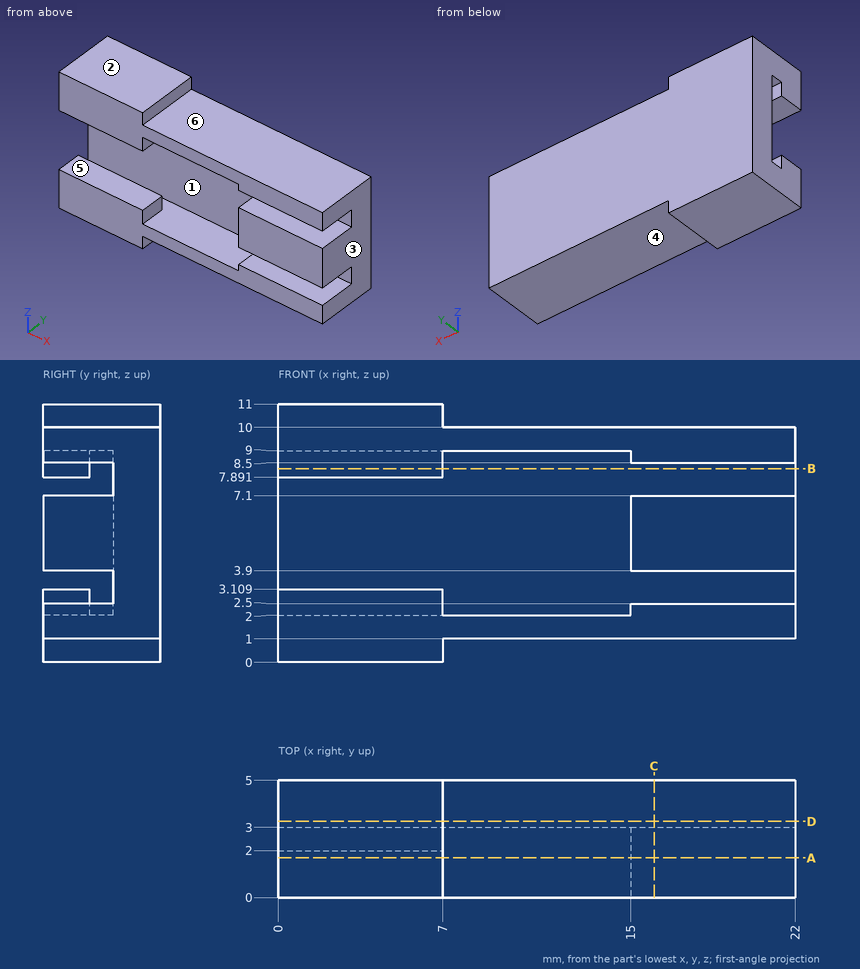
Input: dimensioned drawing with shaded views. Units: mm. Origin: part minimum x, y, z. A direction names the side the tool comes from. Coordinates: 2 decimals unless noted, no trailing zeros. Order: outer loops, then holes, each group sorted by start corner. A loop starts at its lowest first (then second) coordinate and runs counter-clockwise, first axis right, second up. Notation, with made-up numbers: (-10, -25) -> (3, -25) arc R32 cw to (3, 1) -> close; hole circle Ø9 at (31, 56). An arc over 180 degrees is marked (long way). Answer in a Markdown table with one row per item.
Item 1: Section B-B on z = 8.25. Output: boundary loops of the cut face in (x, y), plus the area to 3 significant figures.
Return value:
| item | result |
|---|---|
| outline | (0, 0) -> (7, 0) -> (7, 2) -> (0, 2) -> close; (0, 3) -> (22, 3) -> (22, 5) -> (0, 5) -> close |
| area | 58.0 mm² |
Item 2: Section D-D on y = 3.25. Output: boundary loops of the cut face in (x, z).
Return value:
| item | result |
|---|---|
| outline | (0, 0) -> (7, 0) -> (7, 1) -> (22, 1) -> (22, 10) -> (7, 10) -> (7, 11) -> (0, 11) -> close |
Item 3: Section A-A on y = 1.7. Output: boundary loops of the cut face in (x, z).
Return value:
| item | result |
|---|---|
| outline | (0, 0) -> (7, 0) -> (7, 1) -> (22, 1) -> (22, 2.5) -> (15, 2.5) -> (15, 2) -> (7, 2) -> (7, 3.11) -> (0, 3.11) -> close; (0, 7.89) -> (7, 7.89) -> (7, 9) -> (15, 9) -> (15, 8.5) -> (22, 8.5) -> (22, 10) -> (7, 10) -> (7, 11) -> (0, 11) -> close; (15, 3.9) -> (22, 3.9) -> (22, 7.1) -> (15, 7.1) -> close |
Item 4: Access query for the marked faces 4, 5 and 6. Directions: +Z, -Z, +X, -X, +Y, -Y. A direction counts if a zero-diameter tool reaches every point of the face in a straight line with its end or side. Return the directions, or none.
Return value:
| item | result |
|---|---|
| face 4 | -Z, +X, +Y, -Y |
| face 5 | +X, -X, -Y |
| face 6 | +Z, +X, +Y, -Y |
Item 5: Section C-C on x = 16. Output: boundary loops of the cut face in (y, z).
Return value:
| item | result |
|---|---|
| outline | (0, 1) -> (5, 1) -> (5, 10) -> (0, 10) -> (0, 8.5) -> (3, 8.5) -> (3, 7.1) -> (0, 7.1) -> (0, 3.9) -> (3, 3.9) -> (3, 2.5) -> (0, 2.5) -> close |
Item 6: Draft query along Z for the marked faces 1, 2 and 3. Return one class per face: released by +Z, released by -Z, zero draft, split by the parting line, or undercut.
Return value:
| item | result |
|---|---|
| face 1 | undercut |
| face 2 | released by +Z |
| face 3 | zero draft |
Item 7: Contact query for flat-ended pins moving along their axis: P1, Ø2.5, axis at x = 19.5, y = 1.5, coming from the +Z side; P2, Ø1, axis at x = 8, y = 3.5, coming from the -Z side; P3, Ø0.8, axis at y = 2, z = 10.5, coming from the +X side. Output: stop coordinate, or through.
Return value:
| item | result |
|---|---|
| P1 | stops at z = 10 |
| P2 | stops at z = 1 |
| P3 | stops at x = 7 |
Item 8: Ray query, L1, parallel to Z at x = 18, y = 1.7; L2, parallel to X at y = 0.65, z = 8.75; L3, parallel to Z at x = 5, y = 1.85. Return the intervals inside material, ascending.
Return value:
| item | result |
|---|---|
| L1 | z = 1 to 2.5, 3.9 to 7.1, 8.5 to 10 |
| L2 | x = 0 to 7, 15 to 22 |
| L3 | z = 0 to 3.11, 7.89 to 11 |
